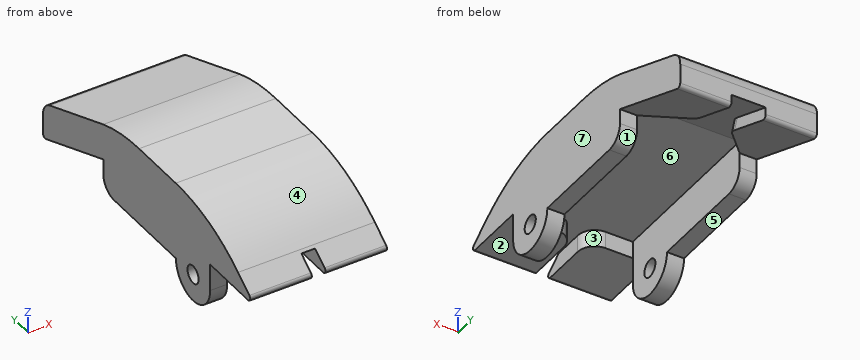
```python
from build123d import *

# Parameters (mm, degrees)
BOSS_EXTRUDE5_DEPTH      = 20
BOSS_EXTRUDE5_DEPTH_BACK = 20
SKETCH6_R                = 2.6000000000000005
SKETCH7_W                = 30.000000000000004
SKETCH7_H                = 21
CUT_EXTRUDE1_DEPTH       = 16
BOSS_EXTRUDE6_DEPTH      = 18
BOSS_EXTRUDE7_DEPTH      = 4
SKETCH12_W               = 4.9999999999999964
SKETCH12_H               = 12.999999999999998
BOSS_EXTRUDE8_DEPTH      = 34
FILLET4_R                = 5
FILLET5_R                = 1
CUT_EXTRUDE3_START       = -15
CUT_EXTRUDE3_DEPTH       = 10
CUT_EXTRUDE4_DEPTH       = 3.360889535
FILLET7_R                = 5
FILLET8_R                = 50


with BuildPart() as part:
    # Sketch6 → Boss-Extrude5 (new, two sides: drawn at the far end of the back side and taken through both)
    with BuildSketch(Plane(origin=(0, 0, 0), x_dir=(0, 0, -1), z_dir=(1, 0, 0)).offset(-BOSS_EXTRUDE5_DEPTH_BACK)):
        with BuildLine():
            Line((-23, -8), (0, -8))
            ThreePointArc((0, -8), (8, 0), (0, 8))
            Line((0, 8), (-13, 7.999999999999998))
            Line((-13, 7.999999999999998), (-13, 42))
            Line((-13, 42), (-9.400224659785392, 42))
            Line((-9.400224659785392, 42), (1.4279133192728315, 70.2082638402405))
            Line((1.4279133192728315, 70.2082638402405), (-9.283536617097441, 70.2082638402405))
            Line((-9.283536617097441, 70.2082638402405), (-20.111674596155662, 42))
            Line((-20.111674596155662, 42), (-23, 42))
            Line((-23, 42), (-23, -8))
        make_face()
        Circle(SKETCH6_R, mode=Mode.SUBTRACT)
    extrude(amount=BOSS_EXTRUDE5_DEPTH + BOSS_EXTRUDE5_DEPTH_BACK)

    # Sketch7 → Cut-Extrude1 (cut)
    with BuildSketch(Plane(origin=(0, 8, 1.07e-15), x_dir=(1, 0, 0), z_dir=(0, 1, 0))):
        with Locations((0, -2.4999999999999982)):
            Rectangle(SKETCH7_W, SKETCH7_H)
    extrude(amount=-CUT_EXTRUDE1_DEPTH, mode=Mode.SUBTRACT)

    # Sketch9 → Boss-Extrude6 (add)
    with BuildSketch(Plane(origin=(20, 0, 0), x_dir=(0, 0, -1), z_dir=(1, 0, 0))):
        Polygon((-8, -8), (-7.9999999999999964, -28.890618944469697), (-23, -8), align=None)
    boss_extrude6 = extrude(amount=-BOSS_EXTRUDE6_DEPTH)

    # Mirror1: Boss-Extrude6 across plane
    add(boss_extrude6.mirror(Plane(origin=(0, 0, 0), x_dir=(0, 0, 1), z_dir=(1, 0, 0))))

    # Sketch10 → Boss-Extrude7 (add)
    with BuildSketch(Plane.ZY.offset(-2)):
        Polygon((23, -8), (13, -8), (13.000000000000004, -21.927079296313124), align=None)
    extrude(amount=BOSS_EXTRUDE7_DEPTH)

    # Sketch12 → Boss-Extrude8 (add)
    with BuildSketch(Plane(origin=(0, 8, 1.07e-15), x_dir=(1, 0, 0), z_dir=(0, 1, 1.3e-16))):
        with Locations((17.5, -6.499999999999999)):
            Rectangle(SKETCH12_W, SKETCH12_H)
    boss_extrude8 = extrude(amount=BOSS_EXTRUDE8_DEPTH)

    # Mirror2: Boss-Extrude8 across plane
    add(boss_extrude8.mirror(Plane(origin=(0, 0, 0), x_dir=(0, 0, 1), z_dir=(1, 0, 0))))

    # Fillet4
    fillet4_edges = [part.edges().sort_by_distance(p)[0] for p in [
        (2, -8, 10.5),
        (-2, -8, 10.5),
    ]]
    fillet(fillet4_edges, radius=FILLET4_R)

    # Fillet5
    fillet5_edges = [part.edges().sort_by_distance(p)[0] for p in [
        (0, 70.2082638402405, -1.4279133192728315),
        (11, -28.890618944469697, 7.9999999999999964),
        (-11, -28.890618944469697, 7.9999999999999964),
    ]]
    fillet(fillet5_edges, radius=FILLET5_R)

    # Sketch13 → Cut-Extrude3 (cut)
    with BuildSketch(Plane(origin=(20, 0, 0), x_dir=(0, 0, -1), z_dir=(1, 0, 0)).offset(CUT_EXTRUDE3_START)):
        Polygon((1.4279133192728315, 70.2082638402405), (-9.400224659785392, 42), (-13.00022465978539, 42), (-2.172086680727171, 70.2082638402405), align=None)
    extrude(amount=-CUT_EXTRUDE3_DEPTH, mode=Mode.SUBTRACT)

    # Sketch14 → Cut-Extrude4 (cut)
    with BuildSketch(Plane(origin=(0, 8.538947678230453, 22.2447192205509), x_dir=(-1, 0, 0), z_dir=(0, -0.3583679495452972, -0.9335804264972031))):
        Polygon((-15.000000000000004, 35.8416386762901), (-5.000000000000001, 48.794944027775955), (-5.000000000000001, 35.8416386762901), (-5.000000000000001, 34.55159456879367), (-15.000000000000004, 34.55159456879367), align=None)
    cut_extrude4 = extrude(amount=-CUT_EXTRUDE4_DEPTH, mode=Mode.SUBTRACT)

    # Mirror3: Cut-Extrude4 across plane
    add(cut_extrude4.mirror(Plane(origin=(0, 0, 0), x_dir=(0, 0, 1), z_dir=(1, 0, 0))), mode=Mode.SUBTRACT)

    # Fillet7
    fillet7_edges = [part.edges().sort_by_distance(p)[0] for p in [
        (17.5, 42, 5.6e-15),
        (-17.5, 42, 5.6e-15),
        (0, 70.2082638402405, 9.283536617097441),
        (5.000000000000001, 54.695169880241785, 6.3270055238869265),
        (-5.000000000000001, 54.695169880241785, 6.3270055238869265),
    ]]
    fillet(fillet7_edges, radius=FILLET7_R)

    # Fillet8
    # the kernel refuses this fillet: 50 mm, written as the material it takes off along each edge
    with BuildSketch(Plane(origin=(61.869597916190855, 42, 23), x_dir=(0, 0, -1), z_dir=(-1, 0, 0))) as fillet8_piece_1:
        with BuildLine():
            CenterArc((50, 16.747839166469827), FILLET8_R, 180, 19.569909983271373)
            Line((0, 16.747839166469827), (-1, 16.747839166469827))
            Line((-1, 16.747839166469827), (-1, 0))
            Line((-1, 0), (0, -1))
            ThreePointArc((0, -1), (1.444162701922167, -1), (1.946091911921222, -0.33495678332939605))
            Line((1.946091911921222, -0.33495678332939605), (2.888325403844334, 0))
        make_face()
    extrude(amount=123.73919583238171, mode=Mode.SUBTRACT)
    with BuildSketch(Plane(origin=(-60.228570108654466, -8.000000000000004, 23), x_dir=(0, -0.812294131590468, -0.5832480122415225), z_dir=(1, 0, 0))) as fillet8_piece_2:
        with BuildLine():
            CenterArc((FILLET8_R * 0.321828560869, FILLET8_R), FILLET8_R, 234.32068370191269, 35.67931629808726)
            Line((-FILLET8_R * 0.261419451372, FILLET8_R * 0.18770586841), (-FILLET8_R * 0.273084411617, FILLET8_R * 0.171459985778))
            Line((-FILLET8_R * 0.273084411617, FILLET8_R * 0.171459985778), (-FILLET8_R * 0.00643657121738, -FILLET8_R * 0.02))
            Line((-FILLET8_R * 0.00643657121738, -FILLET8_R * 0.02), (FILLET8_R * 0.321828560869, -FILLET8_R * 0.02))
            Line((FILLET8_R * 0.321828560869, -FILLET8_R * 0.02), (FILLET8_R * 0.321828560869, 5e-16))
        make_face()
    extrude(amount=120.45714021730896, mode=Mode.SUBTRACT)


solid = part.part
```
The listing builds one solid part. Answer for the finished solid, in the listing's coordinates (mm). Face numbers are marked on the shaded views. A direction names the side the tool comes from. Give positions to 0.01 mm unless a question says otherwise; leave off trailing zeros. Order: outer loops, then holes, each group sorted by start corner. A loop starts at its lowest first (then second) coordinate and runs counter-clockwise, first axis right, second up. Notation, with made-up numbers: (-12.5, -25) -> (10.5, -25) arc R18 ccw to (10.5, -14) -> close; hole circle Ø4 at (23.5, 79). An arc over 180 degrees is marked (long way). Answer as a JSON object with one key per item and string values. Group by question number.
Item 1: Consider L1, parallel to X at y = 7, z = 0.5; L2, parallel to Z at x = -18.4, y = 0; L3, parallel to Z at x = 18, y = 25. Determine where each line is inside the solid, lowest interval first. Write a range as from..to.
Item 2: The part is cut by section D-D on y = 16.5. Write down the section's boundary in (x, z).
Item 3: Determine the mould class of the marked faces 5, 6 and 7 for opening direction X: pulls with the +X half, pulls with the -X half, needs draft (parallel to the pull), parting line crosses it, or undercut.
Item 4: A tool of negligible diameter and unlimited length cuts with its end or side. For the marked faces 1, 2, 3 and 4, from which of +Z, -Z, +X, -X, +Y, -Y can it reach the whole face along a straight path? Write none if from no direction.
Item 5: Flat-ended cylindrical pins translate along their axes: pin 1 (3 mm diameter, centred on x = 15.5, y = 40, fed in from -Z); pin 2 (2.5 mm diameter, centred on x = 17.5, z = 4, fed in from -Y); pin 3 (2.5 mm diameter, centred on x = 12, z = 10, fed in from +Y). Find the tip coordinate at first contact, or state that the pin passes through.
Item 6: The part is cut by section A-A on x = 17. Write down the section's boundary in (y, z).
Item 7: The part is cut by section B-B on y = 0. Write down the section's boundary in (x, z).
Result set:
{
 "1": {"L1": "-20..-15, 15..20", "L2": "-8..-2.6, 2.6..22.34", "L3": "0..23"},
 "2": {"outline": "(-20, 0) -> (-15, 0) -> (-15, 13) -> (15, 13) -> (15, 0) -> (20, 0) -> (20, 23) -> (-20, 23) -> close"},
 "3": {"face 5": "needs draft", "face 6": "undercut", "face 7": "pulls with the +X half"},
 "4": {"face 1": "-Z, +X, -X", "face 2": "-Z, +X, -X, -Y", "face 3": "-Z", "face 4": "+Z, +X, -X, -Y"},
 "5": {"pin 1": "z = 0.23", "pin 2": "y = -8", "pin 3": "y = 69.28"},
 "6": {"outline": "(-26.37, 9.81) arc R1 ccw to (-25.78, 8) -> (-8, 8) -> (-8, 0) arc R8 ccw to (8, 0) -> (37, 0) arc R5 ccw to (42, 5) -> (42, 9.4) -> (68.85, -0.91) arc R1 ccw to (70.21, 0.03) -> (70.21, 5.85) arc R5 ccw to (67, 10.52) -> (42, 20.11) arc R50 ccw to (25.25, 23) -> (8.09, 23) arc R50 ccw to (-21.07, 13.61) -> close; hole circle Ø5.2 at (0, 0)"},
 "7": {"outline": "(-20, -8) -> (-15, -8) -> (-15, -2.6) -> (-20, -2.6) -> close; (-20, 2.6) -> (-15, 2.6) -> (-15, 13) -> (15, 13) -> (15, 2.6) -> (20, 2.6) -> (20, 22.34) -> (-20, 22.34) -> close; (15, -8) -> (20, -8) -> (20, -2.6) -> (15, -2.6) -> close"}
}
